```python
from build123d import *

# Parameters (mm, degrees)
SKETCH1_W            = 172.72
SKETCH1_H            = 99.695
BOSS_EXTRUDE1_DEPTH  = 38.1
SKETCH2_W            = 162.56
SKETCH2_H            = 89.535
CUT_EXTRUDE1_DEPTH   = 31.75
SKETCH3_W            = 6.35
SKETCH3_H            = 6.35
BOSS_EXTRUDE2_DEPTH  = 26.67
SKETCH7_R            = 1.5875
CUT_EXTRUDE3_DEPTH   = 26.67
SKETCH8_W            = 19.558
SKETCH8_H            = 13.208
CUT_EXTRUDE4_DEPTH   = 5.08
SKETCH9_R            = 1.7145
CUT_EXTRUDE6_DEPTH   = 3.4544
SKETCH11_W           = 6.2992
SKETCH11_H           = 12.192
CUT_EXTRUDE7_DEPTH   = 1.6256
SKETCH14_W           = 6.2992
SKETCH14_H           = 3.556
BOSS_EXTRUDE3_DEPTH  = 2.4384
SKETCH22_W           = 3.429
SKETCH22_H           = 10.8585
CUT_EXTRUDE8_DEPTH   = 2.54
BOSS_EXTRUDE16_DEPTH = 2.54
BOSS_EXTRUDE18_DEPTH = 2.54
SKETCH28_W           = 2.54
SKETCH28_H           = 6.096
BOSS_EXTRUDE19_DEPTH = 1.2065
SKETCH29_W           = 2.54
SKETCH29_H           = 6.096
BOSS_EXTRUDE20_DEPTH = 1.2065
CUT_EXTRUDE12_DEPTH  = 7.0485
SKETCH33_W           = 172.72
SKETCH33_H           = 2.54
CUT_EXTRUDE13_DEPTH  = 138.29075943
SKETCH36_W           = 172.72
SKETCH36_H           = 46.9646
BOSS_EXTRUDE21_DEPTH = 12.827
CUT_EXTRUDE14_DEPTH  = 187.167326417
SKETCH41_W           = 9.8425
SKETCH41_H           = 5.7658
BOSS_EXTRUDE22_DEPTH = 12.827
SKETCH42_R           = 2.2225
CUT_EXTRUDE15_DEPTH  = 106.864708266
SKETCH44_W           = 8.6614
SKETCH44_H           = 5.08
BOSS_EXTRUDE24_DEPTH = 10.541
SKETCH46_W           = 1.524
SKETCH46_H           = 10.541
BOSS_EXTRUDE25_DEPTH = 5.6134
SKETCH48_W           = 5.6134
SKETCH48_H           = 1.905
BOSS_EXTRUDE26_DEPTH = 1.27
SKETCH49_W           = 5.6134
SKETCH49_H           = 1.905
BOSS_EXTRUDE27_DEPTH = 1.27
SKETCH50_W           = 5.6134
SKETCH50_H           = 1.905
BOSS_EXTRUDE28_DEPTH = 1.27
SKETCH51_W           = 5.6134
SKETCH51_H           = 1.905
BOSS_EXTRUDE29_DEPTH = 1.27
SKETCH52_W           = 5.6134
SKETCH52_H           = 1.905
BOSS_EXTRUDE30_DEPTH = 1.27
SKETCH53_W           = 5.6134
SKETCH53_H           = 1.905
BOSS_EXTRUDE31_DEPTH = 1.27
SKETCH54_W           = 5.6134
SKETCH54_H           = 1.905
BOSS_EXTRUDE32_DEPTH = 1.27
SKETCH55_W           = 5.6134
SKETCH55_H           = 1.905
BOSS_EXTRUDE33_DEPTH = 1.27
SKETCH56_W           = 5.6134
SKETCH56_H           = 1.905
BOSS_EXTRUDE34_DEPTH = 1.27
SKETCH57_W           = 5.6134
SKETCH57_H           = 1.905
BOSS_EXTRUDE35_DEPTH = 1.27
SKETCH58_W           = 5.6134
SKETCH58_H           = 1.905
BOSS_EXTRUDE36_DEPTH = 1.27
SKETCH59_W           = 5.6134
SKETCH59_H           = 1.905
BOSS_EXTRUDE37_DEPTH = 1.27


with BuildPart() as part:
    # Sketch1 → Boss-Extrude1 (new body)
    with BuildSketch(Plane(origin=(0, 0, 0), x_dir=(1, 0, 0), z_dir=(0, 1, 0))):
        Rectangle(SKETCH1_W, SKETCH1_H)
    extrude(amount=BOSS_EXTRUDE1_DEPTH)

    # Sketch2 → Cut-Extrude1 (cut)
    with BuildSketch(Plane.XZ):
        Rectangle(SKETCH2_W, SKETCH2_H)
    extrude(amount=-CUT_EXTRUDE1_DEPTH, mode=Mode.SUBTRACT)

    # Sketch3 → Boss-Extrude2 (add)
    with BuildSketch(Plane.XZ.offset(-31.75)):
        with Locations((-78.105, 41.5925)):
            Rectangle(SKETCH3_W, SKETCH3_H)
        with Locations((78.105, -41.5925)):
            Rectangle(SKETCH3_W, SKETCH3_H)
    extrude(amount=BOSS_EXTRUDE2_DEPTH)

    # Sketch7 → Cut-Extrude3 (cut)
    with BuildSketch(Plane.XZ.offset(-5.08)):
        with Locations(Location((-78.105, 41.5925, 0), (0, 0, 270))):
            Circle(SKETCH7_R)
        with Locations(Location((78.105, -41.5925, 0), (0, 0, 270))):
            Circle(SKETCH7_R)
    extrude(amount=-CUT_EXTRUDE3_DEPTH, mode=Mode.SUBTRACT)

    # Sketch8 → Cut-Extrude4 (cut)
    with BuildSketch(Plane.XY.offset(49.8475)):
        with Locations((35.306, 16.129)):
            Rectangle(SKETCH8_W, SKETCH8_H)
    extrude(amount=-CUT_EXTRUDE4_DEPTH, mode=Mode.SUBTRACT)

    # Sketch9 → Cut-Extrude6 (cut)
    with BuildSketch(Plane.XY.offset(49.8475)):
        with Locations((6.477, 16.129)):
            Circle(SKETCH9_R)
    extrude(amount=-CUT_EXTRUDE6_DEPTH, mode=Mode.SUBTRACT)

    # Sketch11 → Cut-Extrude7 (cut)
    with BuildSketch(Plane(origin=(0, 0, 44.7675), x_dir=(-1, 0, 0), z_dir=(0, 0, -1))):
        with Locations((-6.477, 19.177)):
            Rectangle(SKETCH11_W, SKETCH11_H)
    extrude(amount=-CUT_EXTRUDE7_DEPTH, mode=Mode.SUBTRACT)

    # Sketch14 → Boss-Extrude3 (add)
    with BuildSketch(Plane(origin=(0, 0, 44.7675), x_dir=(-1, 0, 0), z_dir=(0, 0, -1))):
        Polygon((-9.6266, 9.525), (-9.6266, 13.081), (-9.6266, 19.177), (-13.1826, 19.177), (-13.1826, 9.525), align=None)
        with Locations((-6.477, 11.303)):
            Rectangle(SKETCH14_W, SKETCH14_H)
        Polygon((-3.3274, 19.177), (-3.3274, 13.081), (-3.3274, 9.525), (0.2286, 9.525), (0.2286, 19.177), align=None)
    extrude(amount=BOSS_EXTRUDE3_DEPTH)

    # Sketch22 → Cut-Extrude8 (cut)
    with BuildSketch(Plane(origin=(0, 0, 46.3931), x_dir=(-1, 0, 0), z_dir=(0, 0, -1))):
        with Locations((-6.477, 19.84375)):
            Rectangle(SKETCH22_W, SKETCH22_H)
    extrude(amount=-CUT_EXTRUDE8_DEPTH, mode=Mode.SUBTRACT)

    # Sketch25 → Boss-Extrude16 (add)
    with BuildSketch(Plane(origin=(0, 0, 42.3291), x_dir=(-1, 0, 0), z_dir=(0, 0, -1))):
        Polygon((-9.9441, 13.081), (-9.6266, 13.081), (-9.6266, 19.177), (-11.4046, 19.177), (-11.4046, 13.081), align=None)
        Polygon((-3.3274, 19.177), (-3.3274, 13.081), (-3.0734, 13.081), (-3.0099, 13.081), (-1.5494, 13.081), (-1.5494, 19.177), align=None)
    extrude(amount=BOSS_EXTRUDE16_DEPTH)

    # Sketch25<7> → Boss-Extrude18 (add)
    with BuildSketch(Plane(origin=(0, 0, 42.3291), x_dir=(-1, 0, 0), z_dir=(0, 0, -1))):
        Polygon((-8.4201, 11.811), (-8.4201, 13.081), (-9.6266, 13.081), (-9.9441, 13.081), (-9.9441, 11.811), align=None)
        Polygon((-3.3274, 13.081), (-4.5339, 13.081), (-4.5339, 11.811), (-3.0099, 11.811), (-3.0099, 13.081), (-3.0734, 13.081), align=None)
    extrude(amount=BOSS_EXTRUDE18_DEPTH)

    # Sketch28 → Boss-Extrude19 (add)
    with BuildSketch(Plane(origin=(3.3274, 0, 0), x_dir=(0, 0, -1), z_dir=(1, 0, 0))):
        with Locations((-41.0591, 16.129)):
            Rectangle(SKETCH28_W, SKETCH28_H)
    extrude(amount=BOSS_EXTRUDE19_DEPTH)

    # Sketch29 → Boss-Extrude20 (add)
    with BuildSketch(Plane.ZY.offset(-9.6266)):
        with Locations((41.0591, 16.129)):
            Rectangle(SKETCH29_W, SKETCH29_H)
    extrude(amount=BOSS_EXTRUDE20_DEPTH)

    # Sketch30 → Cut-Extrude12 (cut)
    with BuildSketch(Plane(origin=(9.9441, 0, 0), x_dir=(0, 0, -1), z_dir=(1, 0, 0))):
        Polygon((-39.7891, 13.081), (-42.3291, 11.811), (-39.7891, 11.811), align=None)
    extrude(amount=-CUT_EXTRUDE12_DEPTH, mode=Mode.SUBTRACT)

    # Sketch33 → Cut-Extrude13 (cut, through all)
    with BuildSketch(Plane.XY.offset(49.8475)):
        with Locations((0, 36.83)):
            Rectangle(SKETCH33_W, SKETCH33_H)
    extrude(amount=-CUT_EXTRUDE13_DEPTH, mode=Mode.SUBTRACT)

    # Sketch36 → Boss-Extrude21 (add)
    with BuildSketch(Plane(origin=(0, 35.56, 0), x_dir=(1, 0, 0), z_dir=(0, 1, 0))):
        with Locations((0, 26.3652)):
            Rectangle(SKETCH36_W, SKETCH36_H)
        with Locations((0, -26.3652)):
            Rectangle(SKETCH36_W, SKETCH36_H)
    extrude(amount=BOSS_EXTRUDE21_DEPTH)

    # Sketch37 → Cut-Extrude14 (cut, through all)
    with BuildSketch(Plane.ZY.offset(86.36)):
        Polygon((-49.8475, 35.56), (-49.8475, 48.387), (-2.8829, 48.387), align=None)
        Polygon((2.8829, 48.387), (49.8475, 35.56), (49.8475, 48.387), align=None)
    extrude(amount=-CUT_EXTRUDE14_DEPTH, mode=Mode.SUBTRACT)

    # Sketch41 → Boss-Extrude22 (add, through all)
    with BuildSketch(Plane(origin=(0, 35.56, 0), x_dir=(1, 0, 0), z_dir=(0, 1, 0))):
        with Locations((-81.43875, 0)):
            Rectangle(SKETCH41_W, SKETCH41_H)
        with Locations((81.43875, 0)):
            Rectangle(SKETCH41_W, SKETCH41_H)
    extrude(amount=BOSS_EXTRUDE22_DEPTH)

    # Sketch42 → Cut-Extrude15 (cut, through all)
    with BuildSketch(Plane(origin=(0, 35.56, 0), x_dir=(1, 0, 0), z_dir=(0, 1, 0))):
        with Locations(Location((-63.8175, 0, 0), (0, 0, 270))):
            Circle(SKETCH42_R)
        with Locations(Location((63.8175, 0, 0), (0, 0, 270))):
            Circle(SKETCH42_R)
        with Locations(Location((-38.4175, 0, 0), (0, 0, 270))):
            Circle(SKETCH42_R)
        with Locations(Location((-13.0175, 0, 0), (0, 0, 270))):
            Circle(SKETCH42_R)
        with Locations(Location((12.3825, 0, 0), (0, 0, 270))):
            Circle(SKETCH42_R)
        with Locations(Location((37.7825, 0, 0), (0, 0, 270))):
            Circle(SKETCH42_R)
    extrude(amount=-CUT_EXTRUDE15_DEPTH, mode=Mode.SUBTRACT)

    # Sketch44 → Boss-Extrude24 (add)
    with BuildSketch(Plane(origin=(0, 31.75, 0), x_dir=(-1, 0, 0), z_dir=(0, -1, 0))):
        with Locations((38.4175, -4.7625)):
            Rectangle(SKETCH44_W, SKETCH44_H)
        with Locations((63.8175, -4.7625)):
            Rectangle(SKETCH44_W, SKETCH44_H)
        with Locations((13.0175, -4.7625)):
            Rectangle(SKETCH44_W, SKETCH44_H)
        with Locations((-12.3825, -4.7625)):
            Rectangle(SKETCH44_W, SKETCH44_H)
        with Locations((-37.7825, -4.7625)):
            Rectangle(SKETCH44_W, SKETCH44_H)
        with Locations((-63.9445, -4.7625)):
            Rectangle(SKETCH44_W, SKETCH44_H)
    extrude(amount=BOSS_EXTRUDE24_DEPTH)

    # Sketch46 → Boss-Extrude25 (add)
    with BuildSketch(Plane(origin=(0, 0, 2.2225), x_dir=(-1, 0, 0), z_dir=(0, 0, -1))):
        with Locations((67.3862, 26.4795)):
            Rectangle(SKETCH46_W, SKETCH46_H)
        with Locations((41.9862, 26.4795)):
            Rectangle(SKETCH46_W, SKETCH46_H)
        with Locations((60.2488, 26.4795)):
            Rectangle(SKETCH46_W, SKETCH46_H)
        with Locations((34.8488, 26.4795)):
            Rectangle(SKETCH46_W, SKETCH46_H)
        with Locations((16.5862, 26.4795)):
            Rectangle(SKETCH46_W, SKETCH46_H)
        with Locations((9.4488, 26.4795)):
            Rectangle(SKETCH46_W, SKETCH46_H)
        with Locations((-8.8138, 26.4795)):
            Rectangle(SKETCH46_W, SKETCH46_H)
        with Locations((-15.9512, 26.4795)):
            Rectangle(SKETCH46_W, SKETCH46_H)
        with Locations((-34.2138, 26.4795)):
            Rectangle(SKETCH46_W, SKETCH46_H)
        with Locations((-41.3512, 26.4795)):
            Rectangle(SKETCH46_W, SKETCH46_H)
        with Locations((-60.3758, 26.4795)):
            Rectangle(SKETCH46_W, SKETCH46_H)
        with Locations((-67.5132, 26.4795)):
            Rectangle(SKETCH46_W, SKETCH46_H)
    extrude(amount=BOSS_EXTRUDE25_DEPTH)

    # Sketch48 → Boss-Extrude26 (add)
    with BuildSketch(Plane.ZY.offset(-66.7512)):
        with Locations((-0.5842, 22.1615)):
            Rectangle(SKETCH48_W, SKETCH48_H)
    extrude(amount=BOSS_EXTRUDE26_DEPTH)

    # Sketch49 → Boss-Extrude27 (add)
    with BuildSketch(Plane(origin=(61.1378, 0, 0), x_dir=(0, 0, -1), z_dir=(1, 0, 0))):
        with Locations((0.5842, 22.1615)):
            Rectangle(SKETCH49_W, SKETCH49_H)
    extrude(amount=BOSS_EXTRUDE27_DEPTH)

    # Sketch50 → Boss-Extrude28 (add)
    with BuildSketch(Plane.ZY.offset(-40.5892)):
        with Locations((-0.5842, 22.1615)):
            Rectangle(SKETCH50_W, SKETCH50_H)
    extrude(amount=BOSS_EXTRUDE28_DEPTH)

    # Sketch51 → Boss-Extrude29 (add)
    with BuildSketch(Plane(origin=(34.9758, 0, 0), x_dir=(0, 0, -1), z_dir=(1, 0, 0))):
        with Locations((0.5842, 22.1615)):
            Rectangle(SKETCH51_W, SKETCH51_H)
    extrude(amount=BOSS_EXTRUDE29_DEPTH)

    # Sketch52 → Boss-Extrude30 (add)
    with BuildSketch(Plane.ZY.offset(-15.1892)):
        with Locations((-0.5842, 22.1615)):
            Rectangle(SKETCH52_W, SKETCH52_H)
    extrude(amount=BOSS_EXTRUDE30_DEPTH)

    # Sketch53 → Boss-Extrude31 (add)
    with BuildSketch(Plane(origin=(9.5758, 0, 0), x_dir=(0, 0, -1), z_dir=(1, 0, 0))):
        with Locations((0.5842, 22.1615)):
            Rectangle(SKETCH53_W, SKETCH53_H)
    extrude(amount=BOSS_EXTRUDE31_DEPTH)

    # Sketch54 → Boss-Extrude32 (add)
    with BuildSketch(Plane.ZY.offset(10.2108)):
        with Locations((-0.5842, 22.1615)):
            Rectangle(SKETCH54_W, SKETCH54_H)
    extrude(amount=BOSS_EXTRUDE32_DEPTH)

    # Sketch55 → Boss-Extrude33 (add)
    with BuildSketch(Plane(origin=(-15.8242, 0, 0), x_dir=(0, 0, -1), z_dir=(1, 0, 0))):
        with Locations((0.5842, 22.1615)):
            Rectangle(SKETCH55_W, SKETCH55_H)
    extrude(amount=BOSS_EXTRUDE33_DEPTH)

    # Sketch56 → Boss-Extrude34 (add)
    with BuildSketch(Plane.ZY.offset(35.6108)):
        with Locations((-0.5842, 22.1615)):
            Rectangle(SKETCH56_W, SKETCH56_H)
    extrude(amount=BOSS_EXTRUDE34_DEPTH)

    # Sketch57 → Boss-Extrude35 (add)
    with BuildSketch(Plane(origin=(-41.2242, 0, 0), x_dir=(0, 0, -1), z_dir=(1, 0, 0))):
        with Locations((0.5842, 22.1615)):
            Rectangle(SKETCH57_W, SKETCH57_H)
    extrude(amount=BOSS_EXTRUDE35_DEPTH)

    # Sketch58 → Boss-Extrude36 (add)
    with BuildSketch(Plane.ZY.offset(61.0108)):
        with Locations((-0.5842, 22.1615)):
            Rectangle(SKETCH58_W, SKETCH58_H)
    extrude(amount=BOSS_EXTRUDE36_DEPTH)

    # Sketch59 → Boss-Extrude37 (add)
    with BuildSketch(Plane(origin=(-66.6242, 0, 0), x_dir=(0, 0, -1), z_dir=(1, 0, 0))):
        with Locations((0.5842, 22.1615)):
            Rectangle(SKETCH59_W, SKETCH59_H)
    extrude(amount=BOSS_EXTRUDE37_DEPTH)


solid = part.part
```
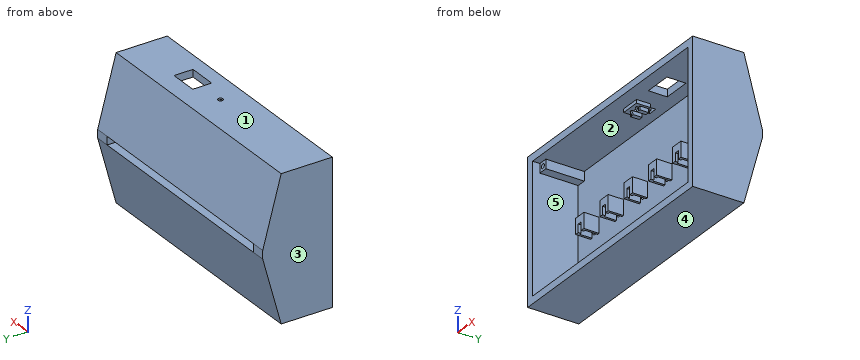
Model file for the job. Use its own axes, mm. Face numbers are marked on the shaded views. A direction names the side the tool comes from. Round coordinates to 2 decimals unless told otherwise and drop trailing zeros. Loops run counter-clockwise (first coordinate to the right, second up) from the corner with the lowest first, then second, coordinate; pieces in that order, holes last. Notation, with made-up numbers: M 25.25,64 L 35.25,64 A5 ccw 35.25,73 Z; hole C -22,-16.5 d5. An arc over 180 degrees is marked long. Put each result on its own line as item: value. Start each with the question number.
Item 1: Cut at D-D (z = 0). Give the number of separate pieces and of enclosed holes in the cut face, then the cut area to 3 significant figures.
Item 2: Drop flat-ended pins along their axis: P1, Ø1, axis at x = -78.5, z = 42, coming from the -Y side; P2, Ø5, axis at x = -29, z = -37.5, coming from the +Y side; P3, Ø4, axis at x = -13.02, z = 0, coming from the -Y side. Give the stop position or say it passes through.
Item 3: Mould opens along X. For the marked faces 1, 2 and 3 say: released by +X, released by -X, zero draft, split by the parting line, or undercut.
Item 4: Cut at A-A (y = 42.5). List the corners of the cut face in (x, z), then the cut area to 3 significant figures.
Item 5: Drill centre lines: line 1 along Z through (x, y) = (8, 4); line 2 along X through (y, z) = (17, 44.5); line 3 along Z through (x, y) = (65, 25). Where is each one in solid material? Low to high.
Item 6: Cut at C-C (z = -35.5). List the corners of the cut face in (x, y), then the cut area to 3 significant figures.
Item 7: Cut at B-B (x = -73). List the corners of the cut face in (y, z).
Item 8: 3-axis set-ups, long thin cutter, end or side, ignore diameter. For the marked faces 4 and 5: which of +Z, -Z, +X, -X, +Y, -Y reach the whole face in a straight line?
Answer block:
1. separate pieces: 7
1. enclosed holes: 0
1. area: 1,350 mm2
2. P1: y = 31.75
2. P2: y = 39.62
2. P3: y = 21.21
3. face 1: zero draft
3. face 2: undercut
3. face 3: released by -X
4. outline: M -86.36,-24.44 L 86.36,-24.44 L 86.36,24.44 L -86.36,24.44 Z; hole M -76.52,-2.88 L 76.52,-2.88 L 76.52,2.88 L -76.52,2.88 Z
4. area: 7,560 mm2
5. line 1: -49.85 to -44.77, 44.77 to 49.85
5. line 2: -86.36 to -74.93, -0.23 to 3.33, 9.63 to 13.18, 81.28 to 86.36
5. line 3: -49.85 to -44.77, 2.22 to 7.3, 44.77 to 49.85
6. outline: M -86.36,0 L -81.28,0 L -81.28,31.75 L 81.28,31.75 L 81.28,0 L 86.36,0 L 86.36,39.48 L -86.36,39.48 Z
6. area: 1,660 mm2
7. outline: M 0,-49.85 L 35.56,-49.85 L 48.39,-2.88 L 35.56,-2.88 L 35.56,2.88 L 48.39,2.88 L 35.56,49.85 L 0,49.85 L 0,44.77 L 31.75,44.77 L 31.75,-44.77 L 0,-44.77 Z
8. face 4: -Z, +X, -X, +Y, -Y
8. face 5: -Y
